Design review of the part shown in the three views and the two pictorial views. Dimensions are in mm from the part's minimum x, y and z. Coordinates: 2 decimals unless noted, no trailing zeros. Write each loop counter-clockwise with the first axis right and the second up, starting at its lowest first coordinate (ties: lowest second). Pieces come first, ordered by that corner, then holes. Notation, with made-up numbers: M 60,-27 L 92,-27 A16 cw 92,-15 Z; hole C 44,-16 d9. An arc over 180 degrees is marked long. Answer as a JSON object with one key per item and string values.
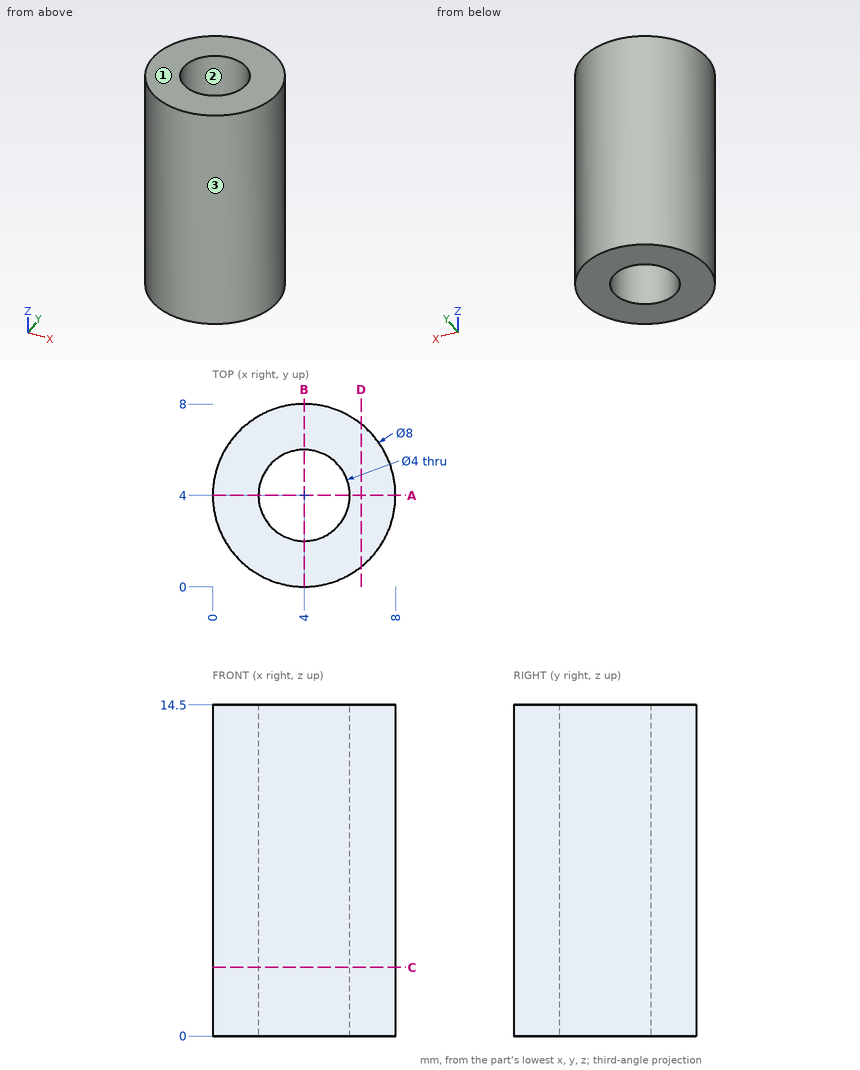
(1) Draft analysis for pull direction X (two halves, no side actions). For the marked faces 1, 2 and 3, state which applies: released by +X, released by -X, zero draft, split by the parting line, or undercut.
Results list:
{"face 1": "zero draft", "face 2": "undercut", "face 3": "split by the parting line"}
(2) Wall thickness on line 1 along Y through (x, z) = (4, 6.5); line 2 along X through (y, z) = (4.5, 11.25); line 3 along X through (y, z) = (2.25, 8): over which ranges is each line inside the solid? List them lowest first. Write a range as from..to.
Results list:
{"line 1": "0..2, 6..8", "line 2": "0.03..2.06, 5.94..7.97", "line 3": "0.4..3.03, 4.97..7.6"}
(3) Add section C-C on z = 3. Give the boundary of the cut face in (x, y), and give its area (3 significant figures).
Results list:
{"outline": "C 4,4 d8; hole C 4,4 d4", "area": "37.7 mm²"}
(4) Add section A-A on y = 4. Give the boundary of the cut face in (x, z).
Results list:
{"outline": "M 0,0 L 2,0 L 2,14.5 L 0,14.5 Z; M 6,0 L 8,0 L 8,14.5 L 6,14.5 Z"}
(5) For pin 1 Ø3 at (x, y) = (5.5, 5.5) entering from -Z; pin 2 Ø1 at (x, z) = (3, 5.5) entering from +Y; pin 3 Ø1.5 at (y, z) = (2.5, 2) entering from -X; pin 4 Ø4 at (y, z) = (1.5, 7.5) entering from -X, all flat-tipped, find the tip position at first contact; note any pin that passes through.
Results list:
{"pin 1": "z = 0", "pin 2": "y = 7.97", "pin 3": "x = 0.07", "pin 4": "x = 0.03"}
(6) Add section D-D on x = 6.5. Give the boundary of the cut face in (y, z).
Results list:
{"outline": "M 0.88,0 L 7.12,0 L 7.12,14.5 L 0.88,14.5 Z"}
